from build123d import *

# Parameters (mm, degrees)
F0_R          = 12.7
F1_DEPTH      = 29.972
F2_R          = 12.7953908212
F3_DEPTH      = 16.764
F3_DEPTH_BACK = 17.018
F5_D          = 12.7
F7_D          = 12.7


with BuildPart() as f1:
    # F0 (on Front) → F1 (new body)
    with BuildSketch(Plane.XZ):
        Circle(F0_R)
    extrude(amount=F1_DEPTH)

    # F2 (on Right) → F3 (join, two sides)
    with BuildSketch(Plane.YZ) as f3_sk:
        with Locations((-14.9844205007, 0)):
            Circle(F2_R)
    extrude(amount=-F3_DEPTH)
    extrude(f3_sk.sketch, amount=F3_DEPTH_BACK)

    # F5 (through all)
    with Locations(Plane(origin=(0, 0, 0), x_dir=(-1, 0, 0), z_dir=(0, 1, 0))):
        with Locations((0, 0)):
            Hole(F5_D / 2)

    # F7 (through all)
    with Locations(Plane(origin=(-16.764, 0, 0), x_dir=(0, -1, 0), z_dir=(-1, 0, 0))):
        with Locations((14.9844205007, 0)):
            Hole(F7_D / 2)


solid = f1.part
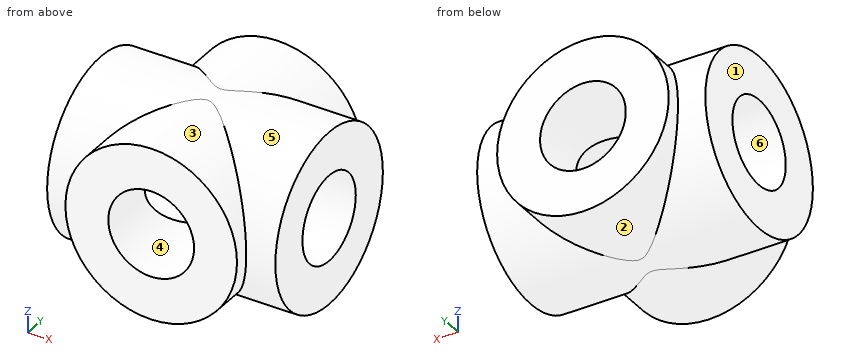
Can you work these out from the model? Positions are in its coordinate system, mm. Face numbers are marked on the shaded views. A direction names the side the tool comes from. Coordinates: 2 decimals unless noted, no trailing zeros. Order: outer loops, then holes, each group sorted by start corner. A loop starts at its lowest first (then second) coordinate and runs counter-clockwise, first axis right, second up. Notation, with made-up numbers: (51.25, -35.75) -> (95.25, -35.75) arc R10 ccw to (95.25, -16.75) -> close; hole circle Ø11 at (8, 6). An arc over 180 degrees is marked (long way). Use one line per item in the form item = value.
Q1. Imagine slicing it at C-C, the plane y = -20. List the corners of the cut face in (x, z) for me.
From the geometry:
outline = (-16.76, -11.77) -> (-4.77, -11.77) arc R12.7 ccw to (4.77, -11.77) -> (17.02, -11.77) -> (17.02, -3.89) -> (5.02, -3.89) arc R6.35 cw to (-5.02, -3.89) -> (-16.76, -3.89) -> close; (-16.76, 3.89) -> (-5.02, 3.89) arc R6.35 cw to (5.02, 3.89) -> (17.02, 3.89) -> (17.02, 11.77) -> (4.77, 11.77) arc R12.7 ccw to (-4.77, 11.77) -> (-16.76, 11.77) -> close
Q2. Imagine slicing it at B-B, the plane x = 2. List the corners of the cut face in (y, z) for me.
From the geometry:
outline = (-29.97, -12.54) -> (-17.52, -12.54) arc R12.8 ccw to (-12.45, -12.54) -> (0, -12.54) -> (0, -6.03) -> (-12.98, -6.03) arc R6.35 cw to (-16.98, -6.03) -> (-29.97, -6.03) -> close; (-29.97, 6.03) -> (-16.98, 6.03) arc R6.35 cw to (-12.98, 6.03) -> (0, 6.03) -> (0, 12.54) -> (-12.45, 12.54) arc R12.8 ccw to (-17.52, 12.54) -> (-29.97, 12.54) -> close
Q3. Imagine slicing it at A-A, the plane z = 0. List the corners of the cut face in (x, y) for me, then the cut area to 3 significant figures.
From the geometry:
outline = (-16.76, -27.78) -> (-12.7, -27.78) -> (-12.7, -29.97) -> (-6.35, -29.97) -> (-6.35, -21.33) -> (-16.76, -21.33) -> close; (-16.76, -8.63) -> (-6.35, -8.63) -> (-6.35, 0) -> (-12.7, 0) -> (-12.7, -2.19) -> (-16.76, -2.19) -> close; (6.35, -29.97) -> (12.7, -29.97) -> (12.7, -27.78) -> (17.02, -27.78) -> (17.02, -21.33) -> (6.35, -21.33) -> close; (6.35, -8.63) -> (17.02, -8.63) -> (17.02, -2.19) -> (12.7, -2.19) -> (12.7, 0) -> (6.35, 0) -> close
area = 327 mm²
Q4. Will these pins go through, and if not, where does the flat tip stop? P1, Ø1, axis at x = 8.5, y = -21, coming from the -Z side; P2, Ø11.5, axis at x = 0, z = 0, coming from the +Y side; P3, Ø1, axis at x = -10.5, y = -15.5, coming from the +Z side; P4, Ø1, axis at x = 7.5, y = -22.5, coming from the +Z side.
From the geometry:
P1 = -11.55
P2 = through
P3 = 12.8
P4 = 10.7
Q5. Which directions (+Z, -Z, +X, -X, +Y, -Y) give clear straight access to the entire face, cutting with the end or side of a thin tool? Please do the marked faces 1, 2 and 3.
From the geometry:
face_1 = +Z, -Z, -X, +Y, -Y
face_2 = +Y
face_3 = -Y
Q6. Imagine slicing it at D-D, the plane y = -6.75. List the corners of the cut face in (x, z) for me.
From the geometry:
outline = (-16.76, -9.79) -> (-8.09, -9.79) arc R12.7 ccw to (8.09, -9.79) -> (17.02, -9.79) -> (17.02, 9.79) -> (8.09, 9.79) arc R12.7 ccw to (-8.09, 9.79) -> (-16.76, 9.79) -> close; hole circle Ø12.7 at (0, 0)
Q7. We'd pull the mould along Y, two halves only. Please class the marked faces 4, 5 and 6: released by +Y, released by -Y, zero draft, split by the parting line, or undercut.
From the geometry:
face_4 = zero draft
face_5 = split by the parting line
face_6 = undercut
Q8. I need wall thicknesses on L1, parallel to Z at x = 0, y = -11; L2, parallel to Y at x = 15.5, z = -0.25; L3, parallel to Z at x = 13, y = -14.75. Which ranges of each line are inside material? Lowest first, please.
From the geometry:
L1 = -12.7 to -6.35, 6.35 to 12.7
L2 = -27.78 to -21.33, -8.64 to -2.19
L3 = -12.79 to -6.35, 6.35 to 12.79
